from build123d import *

# Parameters (mm, degrees)
F0_W     = 113.2934466004
F0_H     = 89.8272059858
F1_DEPTH = 25
F2_R     = 15
F3_T     = -2.5
F5_D     = 5.5


with BuildPart() as f1:
    # F0 (on Top) → F1 (new body)
    with BuildSketch(Plane.XY):
        with Locations((-2.4710707366, -13.6352684349)):
            Rectangle(F0_W, F0_H)
    extrude(amount=F1_DEPTH)

    # F2
    f2_edges = [f1.edges().sort_by_distance(p)[0] for p in [
        (-59.117794, -58.548871, 12.5),
        (54.175653, -58.548871, 12.5),
        (54.175653, 31.278335, 12.5),
        (-59.117794, 31.278335, 12.5),
    ]]
    fillet(f2_edges, radius=F2_R)

    # F3
    f3_openings = [f1.faces().sort_by_distance(p)[0] for p in [
        (-2.471071, -13.635268, 25),
    ]]
    offset(amount=F3_T, openings=f3_openings)

    # F5 (through all)
    with Locations(Plane.XY.offset(2.5)):
        with Locations((-31.6177940369, -6.221665442), (-31.6177940369, -31.221665442), (21.9052377621, -6.221665442), (23.3822059631, -31.221665442)):
            Hole(F5_D / 2)


solid = f1.part
Geometry check sheet. Reference: the model listing, model coordinates, mm. A direction names the side the tool comes from. Give positions to 0.01 mm unless a question says otherwise; leave off trailing zeros. Loops run counter-clockwise (first coordinate to the right, second up) from the corner with the lowest first, then second, coordinate; pieces in that order, holes last.
(1) Release check for a two-part mould opening along Y. For faces 1 (the flat face through (-3, 31.278, 12)), 2 (the cylindrical face through (-54.84, -54.04, 12.68)), 3 (the cylindrical face through (-34.241, -30.396, 1.232)) record: released by +Y, released by -Y, zero draft, split by the parting line, or undercut.
From the geometry:
face 1: released by +Y
face 2: released by -Y
face 3: undercut
(2) Section check A-A on z = 21. Record the cut outline in (x, y), then the cut area to 3 significant figures.
From the geometry:
outline: (-59.12, -43.55) arc R15 ccw to (-44.12, -58.55) - (39.18, -58.55) arc R15 ccw to (54.18, -43.55) - (54.18, 16.28) arc R15 ccw to (39.18, 31.28) - (-44.12, 31.28) arc R15 ccw to (-59.12, 16.28) - close; hole (-56.62, -43.55) arc R12.5 ccw to (-44.12, -56.05) - (39.18, -56.05) arc R12.5 ccw to (51.68, -43.55) - (51.68, 16.28) arc R12.5 ccw to (39.18, 28.78) - (-44.12, 28.78) arc R12.5 ccw to (-56.62, 16.28) - close
area: 932 mm2
(3) Section check B-B on x = -4. Record the cut outline in (y, z).
From the geometry:
outline: (-58.55, 0) - (31.28, 0) - (31.28, 25) - (28.78, 25) - (28.78, 2.5) - (-56.05, 2.5) - (-56.05, 25) - (-58.55, 25) - close
(4) Depth check by flat-ended pin: pin 1 Ø6 at (x, y) = (-23.5, -13.5) entering from +Z; pin 2 Ø4.5 at (x, y) = (-31.62, -31.22) entering from -Z. Enter the tip coordinate at first touch or a pass-through.
From the geometry:
pin 1: stops at z = 2.5
pin 2: passes through
(5) Section check C-C on y = -20.5. Record the cut outline in (x, z), then the cut area to 3 significant figures.
From the geometry:
outline: (-59.12, 0) - (54.18, 0) - (54.18, 25) - (51.68, 25) - (51.68, 2.5) - (-56.62, 2.5) - (-56.62, 25) - (-59.12, 25) - close
area: 396 mm2
(6) Section check D-D on y = -30. Record the cut outline in (x, z), then the cut area to 3 significant figures.
From the geometry:
outline: (-59.12, 0) - (-34.08, 0) - (-34.08, 2.5) - (-56.62, 2.5) - (-56.62, 25) - (-59.12, 25) - close; (-29.15, 0) - (20.92, 0) - (20.92, 2.5) - (-29.15, 2.5) - close; (25.85, 0) - (54.18, 0) - (54.18, 25) - (51.68, 25) - (51.68, 2.5) - (25.85, 2.5) - close
area: 371 mm2
(7) Thickness scan on L1, parallel to X at y = -20, z = 7; L2, parallel to Y at x = 24.5, z = 16.75; L3, parallel to Z at x = -14.5, y = -43.5. Record the ranges inside material, lowest first.
From the geometry:
L1: x = -59.12 to -56.62, 51.68 to 54.18
L2: y = -58.55 to -56.05, 28.78 to 31.28
L3: z = 0 to 2.5
(8) Set-up check for faces 4 (the flat face through (-3, -56.049, 14)), 5 (the cylindrical face through (-34.241, -5.396, 1.232)): record each of +Z, -Z, +X, -X, +Y, -Y from which the full face is reachable in a straight line by a thin tool's end or side.
From the geometry:
face 4: +Z
face 5: +Z, -Z
